Autodesk Inventor part; units mm, degrees
ref_plane "YZ Plane" through (0, 0, 0) normal (1, 0, 0) x (0, 1, 0)
ref_plane "XZ Plane" through (0, 0, 0) normal (0, 1, 0) x (-1, 0, 0)
ref_plane "XY Plane" through (0, 0, 0) normal (0, 0, 1) x (1, 0, 0)
sketch "Sketch2" plane through (0, 0, 0) normal (0, 0, 1) x (1, 0, 0)
  line L0 (0, 0) -> (-6.5, 0)
  line L1 (-6.5, 0) -> (-6.5, 12.8)
  line L2 (-6.5, 12.8) -> (0, 12.8)
  line L3 (0, 12.8) -> (0, 0)
  dimension "d0" = 6.5
  dimension "d1" = 12.8
extrude "Extrusion1" add sketch "Sketch2" along normal blind 5.8
sketch "Sketch3" plane through (0, 0, 5.8) normal (0, 0, 1) x (1, 0, 0)
  line L0 (0, 6.4) -> (-6.5, 6.4)
  line L1 (0, 0) -> (0, 12.8)
  circle A0 centre (-1.3, 3.15) radius 1
  circle A1 centre (-1.3, 9.65) radius 1
  dimension "d4" = 6.5
  dimension "d5" = 6.5
  dimension "d6" = 1.3
  dimension "d7" = 2
  dimension "d8" = 12.8
  dimension "d9" = 0
hole "Hole1" at (-1.3, 3.15, 5.8) at (-1.3, 9.65, 5.8) direction (0, 0, -1) diameter 2 end through all
sketch "Sketch4" plane through (-6.5, 0, 0) normal (-1, 0, 0) x (0, 0, 1)
  line L0 (0, 6.4) -> (6.5, 6.4)
  line L1 (0, 0) -> (5.8, 0)
  line L2 (2.9, 6.4) -> (2.9, 4.12) construction
  line L3 (2.9, 4.12) -> (0.2636, 4.12) construction
  line L4 (0.2636, 4.12) -> (5.5364, 4.12)
  line L5 (4.8, 4.32) -> (1, 4.32)
  line L6 (1, 4.32) -> (1, 3.92)
  line L7 (1, 3.92) -> (4.8, 3.92)
  line L8 (4.8, 3.92) -> (4.8, 4.32)
  line L9 (4.8, 4.32) -> (1, 3.92) construction
  line L10 (1, 4.32) -> (4.8, 3.92) construction
  dimension "d17" = 6.5
  dimension "d18" = 6.4
  dimension "d19" = 2.28
  dimension "d20" = 2.6364
  dimension "d21" = 5.2727
  dimension "d22" = 3.8
  dimension "d23" = 0.4
extrude "Extrusion2" add sketch "Sketch4" along normal blind 0.5
sketch "Sketch5" plane through (-6.5, 3.92, 4.8) normal (0, 0, 1) x (1, 0, 0)
  line L0 (-0.5, 0) -> (-0.5, 0.4)
  line L1 (0, 0) -> (-0.5, 0)
  arc A0 (-0.5, 0.4) -> (-0.5, 0) centre (-0.4899, 0.2) ccw
  point P0 (6.5, -3.92)
extrude "Extrusion3" add sketch "Sketch5" against normal up to surface (3.8 mm away)
chamfer "Chamfer1" distance 0.1 angle 45 10 edges at (-6.5, 0, 2.9) (-6.5, 6.4, 5.8) (-6.5, 6.4, 0) (-6.5, 12.8, 2.9) (-3.25, 12.8, 5.8) (-3.25, 0, 5.8) (-3.25, 0, 0) (-3.25, 12.8, 0) (-1.3, 4.15, 5.8) (-1.3, 10.65, 5.8)
sketch "Sketch6" plane through (0, 0, 0) normal (0, 0, -1) x (-1, 0, 0)
  line L0 (7.3899, 2.6671) -> (9.3, 13.5)
  line L1 (7.3899, 2.6671) -> (18.3899, 2.6671) construction
  line L2 (6.4, 12.7) -> (6.4, 0.1)
  line L3 (6.4, 1.9264) -> (4.4, 1.9264)
  line L4 (6.4, 1.9264) -> (8.4, 1.9264) construction
  arc A0 (6.4, 1.9264) -> (7.3899, 2.6671) centre (6.4, 2.9582) ccw
  line L5 (9.1477, 13.5) -> (7.2437, 2.7017)
  arc A1 (6.4, 2.0764) -> (7.2437, 2.7017) centre (6.4, 2.9582) ccw
  line L6 (6.4, 2.0764) -> (4.4, 2.0764)
  line L7 (4.4, 2.0764) -> (4.4, 1.9264)
  line L8 (9.3, 13.5) -> (9.1477, 13.5)
  line L9 (0, 0) -> (6.4, 0)
  dimension "d31" = 11
  dimension "d32" = 80
  dimension "d33" = 2
  dimension "d34" = 180
  dimension "d35" = 0.15
  dimension "d36" = 9.3
  dimension "d37" = 13.5
  dimension "d38" = 1.0318
extrude "Extrusion4" add sketch "Sketch6" against normal blind 3.8667
equation "\"d4\" = d0"
equation "\"d8\" = d1"
equation "\"d17\" = d0"
equation "\"d18\" = 0.5 * d1"
equation "\"d20\" = 0.454545 * d2"
equation "\"d21\" = 0.909091 * d2"
equation "\"d39\" = 0.666667 * d2"
properties part number "small-tact-switch" material "ABS Plastic"
The model under review builds one solid part; all positions refer to its coordinate system, in mm. A direction names the side the tool comes from. Round coordinates to 2 decimals unless told otherwise and drop trailing zeros. Loops run counter-clockwise (first coordinate to the right, second up) from the corner with the lowest first, then second, coordinate; pieces in that order, holes last. Notation, with made-up numbers: M 15,68.25 L 45,68.25 A20 cw 45,100.25 Z; hole C 46,53.25 d9. An arc over 180 degrees is marked long. Answer as a JSON object with one key per item and string values.
Item 1: We need section B-B, the plane z = 5.4. State the section outline as (x, y) points.
Check sheet entries:
{"outline": "M -6.5,0.1 L -6.4,0 L 0,0 L 0,12.8 L -6.4,12.8 L -6.5,12.7 Z; hole C -1.3,3.15 d2; hole C -1.3,9.65 d2"}
Item 2: We need section C-C, the plane x = -4. State the section outline as (y, z) points.
Check sheet entries:
{"outline": "M 0,0.1 L 0.1,0 L 12.7,0 L 12.8,0.1 L 12.8,5.7 L 12.7,5.8 L 0.1,5.8 L 0,5.7 Z"}
Item 3: We need section A-A, the plane x = -1.3. State the section outline as (y, z) points.
Check sheet entries:
{"outline": "M 0,0.1 L 0.1,0 L 2.15,0 L 2.15,5.7 L 2.05,5.8 L 0.1,5.8 L 0,5.7 Z; M 4.15,0 L 8.65,0 L 8.65,5.7 L 8.55,5.8 L 4.25,5.8 L 4.15,5.7 Z; M 10.65,0 L 12.7,0 L 12.8,0.1 L 12.8,5.7 L 12.7,5.8 L 10.75,5.8 L 10.65,5.7 Z"}
Item 4: Tool access review of faces 4 (the face through (-3, 12.8, 3)), 5 (the face through (-8, 7, 2)), 6 (the face through (-1.6, 2.196, 2.81)): name each direction out of +Z, -Z, +X, -X, +Y, -Y from which nothing blocks a thin tool from reaching the whole face with its end or side.
Check sheet entries:
{"face 4": "+Z, -Z, +X, +Y", "face 5": "+Z, -Z, +Y", "face 6": "+Z, -Z"}
Item 5: The part is to be moulded in two halves that separate along X. For faces 1 (the face through (-3, 0, 3)), 2 (the face through (-7.1, 2.2, 1.9)), 3 (the face through (-1.6, 8.696, 2.81)), say which applies: +X half, -X half, draft (parallel to the pull), parting line (faces both ways), or undercut.
Check sheet entries:
{"face 1": "draft", "face 2": "-X half", "face 3": "undercut"}
Item 6: We need section D-D, the plane y = 3.15. State the section outline as (x, z) points, and give its area (3 significant figures).
Check sheet entries:
{"outline": "M -7.48,0 L -7.32,0 L -7.32,3.87 L -7.48,3.87 Z; M -6.5,0.1 L -6.4,0 L -2.3,0 L -2.3,5.7 L -2.4,5.8 L -6.4,5.8 L -6.5,5.7 Z; M -0.3,0 L 0,0 L 0,5.8 L -0.2,5.8 L -0.3,5.7 Z", "area": "26.7 mm2"}
Item 7: Clearance check with a flat-ended pin moving along its axis: P1, Ø2, axis at x = -8, y = 7.5, coming from the +Z side. State where the tip first meets the part, or that it passes through.
Check sheet entries:
{"P1": "z = 3.87"}
Item 8: For line 1 along Y through (x, z) = (-1.3, 3.5); line 2 along X through (y, z) = (3.75, 1.1); line 3 along X through (y, z) = (3.15, 2.4), list the stretches that pass through material, from the lowest coordinate up.
Check sheet entries:
{"line 1": "0 to 2.15, 4.15 to 8.65, 10.65 to 12.8", "line 2": "-7.58 to -7.43, -6.5 to -2.1, -0.5 to 0", "line 3": "-7.48 to -7.32, -6.5 to -2.3, -0.3 to 0"}
